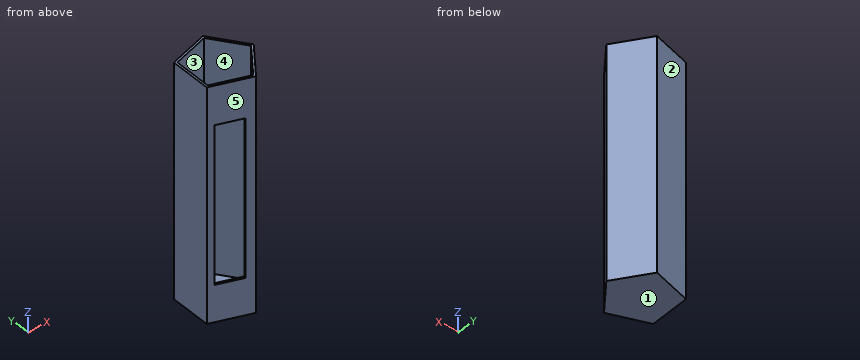
from build123d import *

# Parameters (mm, degrees)
F1_DEPTH = 430
F2_T     = -4
F3_W     = 47.923155129
F3_H     = 290.2228236198
F4_DEPTH = 12.7


with BuildPart() as f1:
    # F0 (on Top) → F1 (new body)
    with BuildSketch(Plane.XY):
        Polygon((17.8408334003, -62.3160021047), (64.7791605856, -2.2890628103), (22.1948896043, 60.9012834855), (-51.0619644336, 39.9281259628), (-53.7529191566, -36.2243445334), align=None)
    extrude(amount=F1_DEPTH)

    # F2
    f2_openings = [f1.faces().sort_by_distance(p)[0] for p in [
        (0, 0, 430),
    ]]
    offset(amount=F2_T, openings=f2_openings)

    # F3 (on face) → F4 (cut)
    with BuildSketch(Plane(origin=(-17.9560428781, -49.270173319, 0), x_dir=(0.9395505585, -0.3424102043, 0), z_dir=(-0.3424102043, -0.9395505585, 0))):
        with Locations((-2.0299293101, 212.9202485085)):
            Rectangle(F3_W, F3_H)
    extrude(amount=-F4_DEPTH, mode=Mode.SUBTRACT)


solid = f1.part
Read the model definition and answer for the solid it produces. Units are mm, in the model's axes. Face numbers are marked on the shaded views. A direction names the side the tool comes from. Round coordinates to 2 decimals unless told otherwise and drop trailing zeros. Write each loop counter-clockwise with the first axis right and the second up, starting at its lowest first coordinate (ties: lowest second). Pieces come first, ordered by that corner, then holes. Notation, with made-up numbers: M 53,26 L 88,26 A7 cw 88,34 Z; hole C 85,-13 d6. An arc over 180 degrees is marked long. Use a Markdown table: item, result.
1) The part is cut by section D-D (y = -21). Write down the section's boundary in (x, z), plus the area to 3 significant figures.
Answers follow:
| item | result |
|---|---|
| outline | M -53.21,0 L 50.15,0 L 50.15,430 L 45.07,430 L 45.07,4 L -49.21,4 L -49.21,430 L -53.21,430 Z |
| area | 4,280 mm2 |
2) The part is cut by section C-C (y = -48). Write down the section's boundary in (x, z).
Answers follow:
| item | result |
|---|---|
| outline | M -21.44,0 L 29.04,0 L 29.04,430 L 23.96,430 L 23.96,4 L -9.76,4 L -9.76,67.81 L -21.44,67.81 Z; M -21.44,358.03 L -9.76,358.03 L -9.76,430 L -21.44,430 Z |
3) The part is cut by section A-A (z = 81.5). Write down the section's boundary in (x, y).
Answers follow:
| item | result |
|---|---|
| outline | M -53.75,-36.22 L -42.38,-40.37 L -41.01,-36.61 L -49.65,-33.46 L -47.17,36.88 L 20.5,56.26 L 59.84,-2.11 L 16.48,-57.56 L 4.02,-53.02 L 2.65,-56.78 L 17.84,-62.32 L 64.78,-2.29 L 22.19,60.9 L -51.06,39.93 Z |
4) The part is cut by section B-B (x = -17.5). Write down the section's boundary in (y, z), plus the area to 3 significant figures.
Answers follow:
| item | result |
|---|---|
| outline | M -49.44,0 L 49.54,0 L 49.54,430 L 45.38,430 L 45.38,4 L -45.18,4 L -45.18,67.81 L -49.44,67.81 Z; M -49.44,358.03 L -45.18,358.03 L -45.18,430 L -49.44,430 Z |
| area | 2,750 mm2 |
5) Flat-ended cylindrical pins translate along their axes: pin 1 (3 mm diameter, centred on x = -34, z = 71, fed in from -Y); pin 2 (12 mm diameter, centred on y = -14, z = 175.5, fed in from +X); pin 3 (5 mm diameter, centred on x = 25, y = -45.5, fed in from -Z); pin 4 (2 mm diameter, centred on x = -15, z = 309.5, fed in from +Y). Find the tip coordinate at first contact, or state that the pin passes through.
Answers follow:
| item | result |
|---|---|
| pin 1 | stops at y = 40.22 |
| pin 2 | stops at x = 60.31 |
| pin 3 | stops at z = 0 |
| pin 4 | stops at y = 50.54 |
6) A tool of negligible diameter and unlimited length cuts with its end or side. For the marked faces 4 and 5, from which of +Z, -Z, +X, -X, +Y, -Y can it reach the whole face along a straight path? Write none if from no direction.
Answers follow:
| item | result |
|---|---|
| face 4 | +Z |
| face 5 | +Z, -Z, -X, -Y |
7) Straight lines are drawn through the part: line 1 along Z through (x, y) = (38, 9); line 2 along Y through (x, z) = (45, 320.5); line 3 along Y through (x, z) = (23.5, 55.5). For each, find the intervals that lie inside material, in ascending order. Write a range as [from, to].
Answers follow:
| item | result |
|---|---|
| line 1 | z = [0, 4] |
| line 2 | y = [-27.58, -21.09], [19.9, 27.06] |
| line 3 | y = [-55.08, -48.59], [51.81, 58.96] |
8) For a pull along Y with two mould halves and no side action, classify the marked faces 1, 2 and 3 as pulls with the +Y half, pulls with the -Y half, needs draft (parallel to the pull), parting line crosses it, or undercut.
Answers follow:
| item | result |
|---|---|
| face 1 | needs draft |
| face 2 | pulls with the +Y half |
| face 3 | undercut |
